Build history of the part. All positions in model axes, mm. A direction names the side the tool comes from. Coordinates: 2 decimals unless noted, no trailing zeros. Write each loop counter-clockwise with the first axis right and the second up, starting at its lowest first coordinate (ties: lowest second). Pieces come first, ordered by that corner, then holes.
```python
from build123d import *

# Parameters (mm, degrees)
F0_R     = 1.5
F1_DEPTH = 12
F3_DEPTH = 8
F5_DEPTH = 16


with BuildPart() as f1:
    # F0 (on Front) → F1 (new body, symmetric)
    with BuildSketch(Plane.XZ):
        with BuildLine():
            ThreePointArc((-21.167, 34.54), (-24.7592769863, 32.2994163957), (-24.3271555139, 28.0877730268))
            Line((-24.3271555139, 28.0877730268), (-1.5800777569, -1.2261134866))
            ThreePointArc((-1.5800777569, -1.2261134866), (0.6732360047, -1.8832825816), (1.9992859745, 0.0534377403))
            Line((1.9992859745, 0.0534377403), (1.181571949, 30.6468754807))
            ThreePointArc((1.181571949, 30.6468754807), (-0.0266148942, 33.4059642289), (-2.817, 34.54))
            Line((-2.817, 34.54), (-21.167, 34.54))
        make_face()
        with Locations((-21.167, 30.54)):
            Circle(F0_R, mode=Mode.SUBTRACT)
        with Locations((-2.817, 30.54)):
            Circle(F0_R, mode=Mode.SUBTRACT)
    extrude(amount=F1_DEPTH, both=True)

    # F2 (on Front) → F3 (cut, symmetric)
    with BuildSketch(Plane.XZ):
        with BuildLine():
            ThreePointArc((-1.5800777569, -1.2261134866), (0.6732360047, -1.8832825816), (1.9992859745, 0.0534377403))
            Line((1.9992859745, 0.0534377403), (1.181571949, 30.6468754807))
            ThreePointArc((1.181571949, 30.6468754807), (-0.0266148942, 33.4059642289), (-2.817, 34.54))
            Line((-2.817, 34.54), (-21.167, 34.54))
            ThreePointArc((-21.167, 34.54), (-24.7592769863, 32.2994163957), (-24.3271555139, 28.0877730268))
            Line((-24.3271555139, 28.0877730268), (-1.5800777569, -1.2261134866))
        make_face()
    extrude(amount=F3_DEPTH, both=True, mode=Mode.SUBTRACT)

    # F4 (on face) → F5 (join)
    with BuildSketch(Plane.XZ.offset(-8)):
        with BuildLine():
            ThreePointArc((-1.5800777569, -1.2261134866), (0.6732360047, -1.8832825816), (1.9992859745, 0.0534377403))
            Line((1.9992859745, 0.0534377403), (1.4575929373, 20.32))
            Line((1.4575929373, 20.32), (-18.2994956552, 20.32))
            Line((-18.2994956552, 20.32), (-1.5800777569, -1.2261134866))
        make_face()
    extrude(amount=F5_DEPTH)


solid = f1.part
```
1. Saw through at C-C on z = 1. List the corners of the cut face in (x, y).
Computed values:
outline: (-3.31, -12) - (1.97, -12) - (1.97, 12) - (-3.31, 12) - close
2. 3-axis set-ups, long thin cutter, end or side, ignore diameter. For faces 1 (the face through (-12, 10, 34.54)), 2 (the face through (-12, 8, 28)): which of +Z, -Z, +X, -X, +Y, -Y reach the whole face in a straight line?
Computed values:
face 1: +Z, +X, -X, +Y, -Y
face 2: +Z, +X, -X
3. Saw through at B-B on y = 2.25. List the corners of the cut face in (x, z), plus the area to 3 significant figures.
Computed values:
outline: (-18.3, 20.32) - (-1.58, -1.23) arc R2 ccw to (2, 0.05) - (1.46, 20.32) - close
area: 253 mm2
4. Flat gauge pins, fed straight in: pin 1 (2 mm diameter, centred on y = -3, z = 5, fed in from -X); pin 2 (1.5 mm diameter, centred on x = -5, y = 3.5, fed in from -Z); pin 3 (6 mm diameter, centred on x = -19, y = 3, fed in from -Z); pin 4 (1.8 mm diameter, centred on x = -2.817, z = 30.54, fed in from -Y). Where does each tip first touch, or does it go through?
Computed values:
pin 1: stops at x = -7.19
pin 2: stops at z = 2.21
pin 3: stops at z = 17.36
pin 4: passes through
5. Saw through at D-D on x = -7.5. List the corners of the cut face in (y, z).
Computed values:
outline: (-12, 6.4) - (12, 6.4) - (12, 34.54) - (8, 34.54) - (8, 20.32) - (-8, 20.32) - (-8, 34.54) - (-12, 34.54) - close
6. Mould opens along Z. For faces 3 (the face through (-3.012, 10.028, 32.027)), 4 (the face through (-24.73, 9.97, 32.36)), 5 (the face through (-9, -12, 21)) say: +Z half, -Z half, draft (parallel to the pull), parting line (faces both ways), or undercut.
Computed values:
face 3: undercut
face 4: parting line
face 5: draft
7. Probe line 1 along X through (y, z) = (-9.65, 30.54); line 2 along Y through (x, z) = (-11, 22.5); line 3 along Z through (x, y) = (-1.5, -2.5). List the from-to ranges inside material, lowest first.
Computed values:
line 1: x = -25.17 to -22.67, -19.67 to -4.32, -1.32 to 1.18
line 2: y = -12 to -8, 8 to 12
line 3: z = -1.32 to 20.32
8. Saw through at A-A on x = -15.75. List the corners of the cut face in (y, z), plus the area to 3 significant figures.
Computed values:
outline: (-12, 17.03) - (12, 17.03) - (12, 34.54) - (8, 34.54) - (8, 20.32) - (-8, 20.32) - (-8, 34.54) - (-12, 34.54) - close
area: 193 mm2
